Part model, mm, in its own coordinate system. A direction names the side the tool comes from. Round coordinates to 2 decimals unless told otherwise and drop trailing zeros. Order: outer loops, then holes, each group sorted by start corner. A loop starts at its lowest first (then second) coordinate and runs counter-clockwise, first axis right, second up. Notation, with made-up numbers: (-37.75, 86) - (-16.75, 86) arc R21 ccw to (-16.75, 118) - close; hole circle Ø9 at (89, -39). An arc over 180 degrees is marked (long way). Answer as a JSON object with one key per item and string values.
Autodesk Inventor part; units mm, degrees
ref_plane "YZ Plane" through (0, 0, 0) normal (1, 0, 0) x (0, 1, 0)
ref_plane "XZ Plane" through (0, 0, 0) normal (0, 1, 0) x (-1, 0, 0)
ref_plane "XY Plane" through (0, 0, 0) normal (0, 0, 1) x (1, 0, 0)
sketch "Sketch8" plane through (0, 0, 0) normal (1, 0, 0) x (0, 1, 0)
  line L0 (0, 0) -> (-50, 0)
  line L1 (-50, 0) -> (-50, -16.325)
  line L2 (-50, -16.325) -> (0, -16.325)
  line L3 (0, -16.325) -> (0, 0)
  dimension "d20" = 50
  dimension "d21" = 16.325
extrude "Extrusion5" add sketch "Sketch8" along normal blind 6
sketch "Sketch9" plane through (0, -50, -16.325) normal (0, -1, 0) x (1, 0, 0)
  circle A0 centre (3, 12.925) radius 1.4
  circle A1 centre (3, 3.4) radius 1
  line L0 (0, 16.325) -> (6, 16.325)
  line L1 (0, 16.325) -> (0, 0)
  line L2 (6, 16.325) -> (6, 0)
  line L3 (0, 0) -> (6, 0)
  line L4 (3, 16.325) -> (3, 0)
  line L5 (0, 8.1625) -> (6, 8.1625)
  dimension "d24" = 2.8
  dimension "d25" = 2
  dimension "d30" = 9.525
  dimension "d31" = 9.525
  dimension "d32" = 0
  dimension "d33" = 0
extrude "Extrusion6" cut sketch "Sketch9" against normal through all contours A0 L4 | L4 A0 | L4 A1 | A1 L4
sketch "Sketch10" plane through (6, 0, 0) normal (1, 0, 0) x (0, 0, -1)
  line L0 (0, 0) -> (0, -50)
  line L1 (0, -50) -> (5.5, -50)
  line L2 (5.5, -50) -> (5.5, -48)
  line L3 (5.5, -48) -> (0, -48)
  line L4 (0, -48) -> (0, -50)
  line L5 (16.325, 0) -> (0, 0)
  line L6 (0, 0) -> (5.5, 0)
  line L7 (5.5, 0) -> (5.5, -2)
  line L8 (5.5, -2) -> (0, -2)
  line L9 (0, -2) -> (0, 0)
  dimension "d36" = 5.5
  dimension "d37" = 2
  dimension "d38" = 2
extrude "Extrusion7" cut sketch "Sketch10" against normal through all
sketch "Sketch11" plane through (6, 0, 0) normal (1, 0, 0) x (0, 0, -1)
  line L0 (0, -2) -> (0, -48)
  line L1 (0, -25) -> (16.325, -25)
  line L2 (16.325, -50) -> (16.325, 0)
  line L3 (5.5, -40) -> (0, -40)
  line L4 (0, -40) -> (0, -10)
  line L5 (0, -10) -> (5.5, -10)
  line L6 (5.5, -10) -> (5.5, -40)
  line L7 (5.5, -40) -> (0, -10) construction
  line L8 (0, -40) -> (5.5, -10) construction
  point P0 (0, 0)
  point P1 (2.75, -25)
  dimension "d41" = 2.75
  dimension "d42" = 30
extrude "Extrusion8" cut sketch "Sketch11" against normal through all
sketch "Sketch12" plane through (6, -48, -5.5) normal (0, -1, 0) x (1, 0, 0)
  circle A0 centre (-3, 2.1) radius 1.4
  circle A1 centre (-3, 2.1) radius 3
  line L0 (-6, 5.5) -> (-6, 0)
  line L1 (0, -10.825) -> (0, 0)
  line L2 (-3, -0.9) -> (-6, -0.9)
  line L3 (-6, -10.825) -> (-6, 0)
  line L4 (0, 0) -> (0, 5.5)
  line L5 (0, 2.1) -> (0, 5.5)
  line L6 (0, 5.5) -> (-6, 5.5)
  line L7 (-6, -0.9) -> (-6, 5.5)
  point P0 (0, -0.9)
extrude "Extrusion9" cut sketch "Sketch12" against normal blind 8 contours L2 L3 L0 A1 | A1 L0 L6 L4
sketch "Sketch13" plane through (0, 0, 0) normal (-1, 0, 0) x (0, 0, 1)
  line L0 (-6.4, -48) -> (-6.4, -40)
  line L1 (-16.325, -50) -> (-6.4, -50)
  line L2 (-6.4, -50) -> (-6.4, -39.4)
  line L3 (-6.4, -39.4) -> (-16.325, -39.4)
  line L4 (-16.325, -39.4) -> (-16.325, -50)
  point P0 (0, 0)
  dimension "d47" = 10.6
extrude "Extrusion10" cut sketch "Sketch13" against normal through all
properties part number "tracks2"
Item 1: Cut at D-D (x = 5.5). Write the cut outline in (y, z) (3 decimals).
Taken from the geometry:
{"outline": "(-50, -6.4) - (-39.4, -6.4) - (-39.4, -16.325) - (0, -16.325) - (0, -5.5) - (-2, -5.5) - (-2, 0) - (-10, 0) - (-10, -5.5) - (-40, -5.5) - (-40, -1.742) - (-48, -1.742) - (-48, -5.5) - (-50, -5.5) - close"}
Item 2: Cut at C-C (z = -15). Write the cut outline in (x, y).
Taken from the geometry:
{"outline": "(0, -39.4) - (6, -39.4) - (6, 0) - (0, 0) - close"}
Item 3: Probe L1, parallel to Y at x = 2.9, z = -5; L2, parallel to Z at x = 3, y = -23 (3 decimals); L3, parallel to Y at x = 0.75, z = -11.5. List the from-to ranges inside material, lowest first. Write a range as from..to.
Taken from the geometry:
{"L1": "-48..-40, -10..-2", "L2": "-16.325..-13.925, -11.925..-5.5", "L3": "-39.4..0"}
Item 4: Tool access for faces 4 (the flat face through (4, -10, -2)), 5 (the flat face through (4, -46, -6.4)), 6 (the flat face through (1, -48, -6)), 7 (the flat face through (3, -1, -5.5)): list every direction of +Z, -Z, +X, -X, +Y, -Y with a clear straight run to the whole face (end or side of a thin tool).
Taken from the geometry:
{"face 4": "+Z, +X, -X", "face 5": "-Z, +X, -X, -Y", "face 6": "-Z, -X", "face 7": "+Z, +X, -X, +Y"}
Item 5: Drop flat-ended pins along their axis: P1, Ø1, axis at x = 4.5, z = -2, coming from the +Y side; P2, Ø1.8, axis at x = 4, y = -28, coming from the +Z side; P3, Ø1.8, axis at x = 3, z = -12.925, coming from the +Y side; P4, Ø1.8, axis at x = 3.5, y = -44.5, coming from the -Z side. Give the stop position or say it passes through.
Taken from the geometry:
{"P1": "y = -2", "P2": "z = -5.5", "P3": "through", "P4": "z = -6.4"}
Item 6: Cut at B-B (y = -24). Write the cut outline in (x, z) (3 decimals), plus the area to 3 significant figures.
Taken from the geometry:
{"outline": "(0, -16.325) - (6, -16.325) - (6, -5.5) - (0, -5.5) - close; hole circle Ø2 at (3, -12.925)", "area": "61.8 mm2"}
Item 7: Two-plate mould, pull along Y, no slides. Class faces 1 (the flat face through (1, -40, -6)), 2 (the flat face through (3.04, -48, -1.85)), 3 (the flat face through (3, -49, -5.5)): pulls with the +Y half, pulls with the -Y half, needs draft (parallel to the pull), parting line crosses it, or undercut.
Taken from the geometry:
{"face 1": "undercut", "face 2": "pulls with the -Y half", "face 3": "needs draft"}
Item 8: Cut at A-A (z = -3.4). Write the cut outline in (x, y), plus the area to 3 significant figures.
Taken from the geometry:
{"outline": "(0, -48) - (1.6, -48) - (1.6, -40) - (0, -40) - close; (0, -10) - (1.6, -10) - (1.6, -2) - (0, -2) - close; (4.4, -48) - (6, -48) - (6, -40) - (4.4, -40) - close; (4.4, -10) - (6, -10) - (6, -2) - (4.4, -2) - close", "area": "51.2 mm2"}
